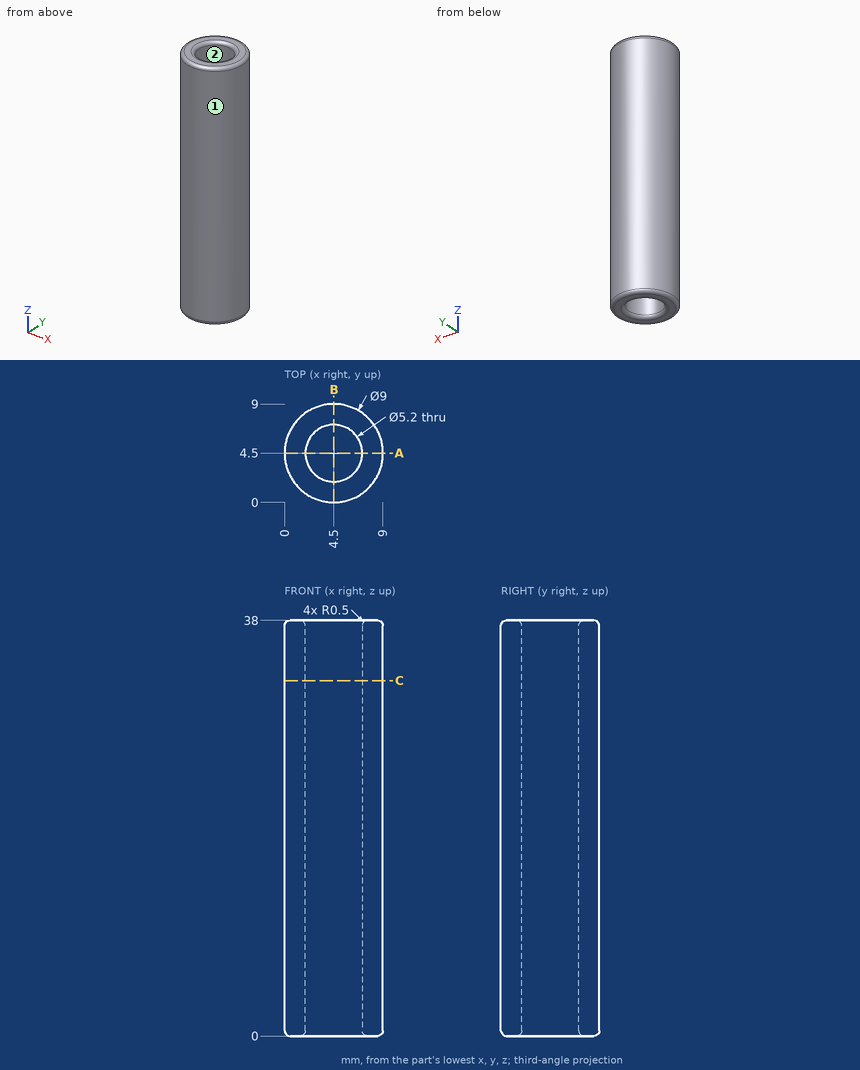
Geometry check sheet. Reference: drawing and pictorial views, mm from the part's lowest x, y, z. Give positions to 0.01 mm unless a question says otherwise; leave off trailing zeros. Write each loop counter-clockwise with the first axis right and the second up, starting at its lowest first coordinate (ties: lowest second). Pieces come first, ordered by that corner, then holes. Notation, with made-up numbers: (17, -1.75) -> (55, -1.75) arc R24 cw to (55, 12.25) -> close; hole circle Ø6 at (80, 71.25). An arc over 180 degrees is marked (long way). One line per question, with ' | ' between items.
Item 1: Sectioned sample at A-A, the plane y = 4.5. Record the boundary of the cut face in (x, z).
Determined:
outline: (0, 0.5) arc R0.5 ccw to (0.5, 0) -> (1.4, 0) arc R0.5 ccw to (1.9, 0.5) -> (1.9, 37.5) arc R0.5 ccw to (1.4, 38) -> (0.5, 38) arc R0.5 ccw to (0, 37.5) -> close; (7.1, 0.5) arc R0.5 ccw to (7.6, 0) -> (8.5, 0) arc R0.5 ccw to (9, 0.5) -> (9, 37.5) arc R0.5 ccw to (8.5, 38) -> (7.6, 38) arc R0.5 ccw to (7.1, 37.5) -> close
Item 2: Draft check along Y on the marked faces 1 and 2. Enter one of: released by +Y, released by -Y, zero draft, split by the parting line, or undercut.
Determined:
face 1: split by the parting line | face 2: undercut
Item 3: Scan lines: line 1 along Y through (x, z) = (4.5, 19); line 2 along X through (y, z) = (2.75, 11); line 3 along Y through (x, z) = (6, 10). Record each from-to range of solid material in increasing order.
Determined:
line 1: 0 to 1.9, 7.1 to 9 | line 2: 0.35 to 2.58, 6.42 to 8.65 | line 3: 0.26 to 2.38, 6.62 to 8.74
Item 4: Depth check by flat-ended pin: pin 1 (1 mm diameter, centred on y = 5.5, z = 21, fed in from +X); pin 2 (1 mm diameter, centred on x = 5.5, y = 5.5, fed in from -Z); pin 3 (1.5 mm diameter, centred on y = 5.5, z = 30, fed in from -X). Enter the tip coordinate at first touch or a pass-through.
Determined:
pin 1: x = 8.97 | pin 2: through | pin 3: x = 0.01
Item 5: Sectioned sample at C-C, the plane z = 32.5. Record the boundary of the cut face in (x, y).
Determined:
outline: circle Ø9 at (4.5, 4.5); hole circle Ø5.2 at (4.5, 4.5)
